Answer from the drawing. Dimensions are ordinates in mm from the lowest x, y and z of the part. A direction names the side the tool comes from. Round coordinates to 2 decimals unless told otherwise and drop trailing zeros. Loops run counter-clockwise (first coordinate to the right, second up) from the corner with the lowest first, then second, coordinate; pieces in that order, holes last. Notation, with made-up numbers: (-4.5, -36.5) - (50.5, -36.5) arc R21 ccw to (50.5, -2.5) - close; hole circle Ø3 at (82, 86). An arc over 180 degrees is marked (long way). Answer as CSV lines item,"result". Start each with the question number.
Q1. Section A-A on z = 1.75 is taken. Write down the section's boundary in (x, y).
Q2. Each of these flat-tipped pins is pushed along its axis until it touches: pin 1 Ø4 at (x, z) = (46, 1) entering from +Y; pin 2 Ø3 at (y, z) = (20.5, 4) entering from -X. Where does it stop, or does it pass through?
Q3. Straight lines are drawn through the part: L1, parallel to Y at x = 26, z = 3.5; L2, parallel to X at y = 14.25, z = 3.5; L3, parallel to X at y = 16.5, z = 2.25. For each, find the intervals that lie inside material, in ascending order. Write a range as [from, to].
Q4. Section B-B on y = 13.5 is taken. Write down the section's boundary in (x, z), then the cut area to 3 significant figures.
Q5. For the marked faces 1 and 2, determine the directions among +Z, -Z, +X, -X, +Y, -Y from which every point of the face is accessible in a straight line to the end or side of a thin tool.
Q6. Section C-C on x = 25 is taken. Write down the section's boundary in (y, z), then the cut area to 3 significant figures.
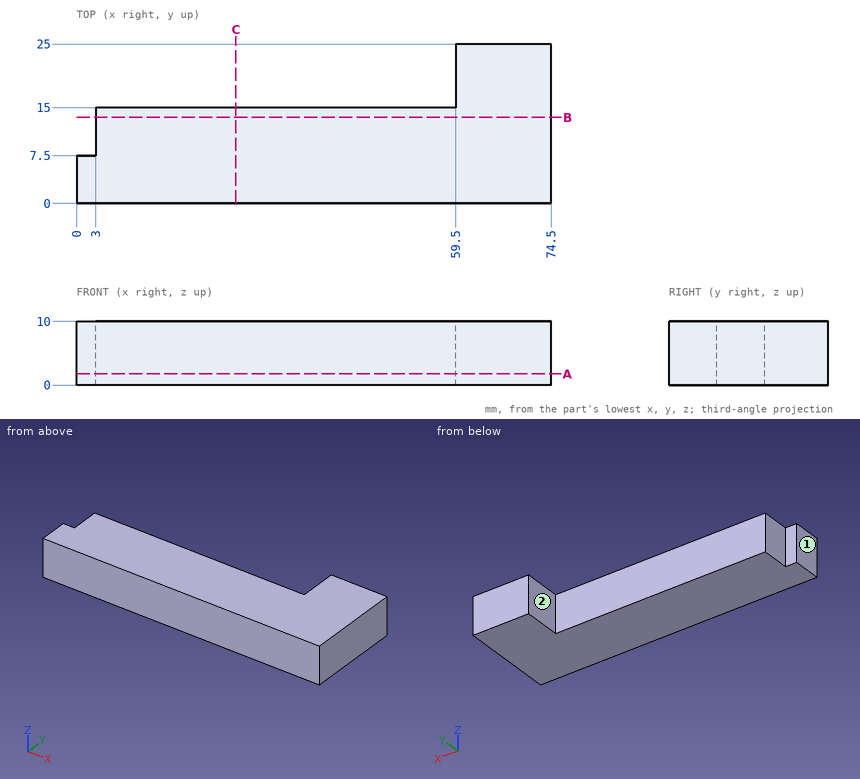
Findings:
1,outline,"(0, 0) - (74.5, 0) - (74.5, 25) - (59.5, 25) - (59.5, 15) - (3, 15) - (3, 7.5) - (0, 7.5) - close"
2,pin 1,"stops at y = 15"
2,pin 2,"stops at x = 59.5"
3,L1,"y = [0, 15]"
3,L2,"x = [3, 74.5]"
3,L3,"x = [59.5, 74.5]"
4,outline,"(3, 0) - (74.5, 0) - (74.5, 10) - (3, 10) - close"
4,area,"715 mm^2"
5,face 1,"+Z, -Z, -X, +Y, -Y"
5,face 2,"+Z, -Z, -X, +Y"
6,outline,"(0, 0) - (15, 0) - (15, 10) - (0, 10) - close"
6,area,"150 mm^2"
